Check sheet for the modelled part. Datum: model origin and axes. Units: mm. Give positions to 0.01 mm unless a question says otherwise; leave off trailing zeros. Loops run counter-clockwise (first coordinate to the right, second up) from the corner with the lowest first, then second, coordinate; pieces in that order, holes last. Notation, with made-up numbers: M 45.25,-23.5 L 102.25,-23.5 A29 cw 102.25,2.5 Z; hole C 85.25,37 d7. An arc over 180 degrees is marked long. Write each question's results on one line, items separated by ' | '. Start each with the question number.
1. Sectioned sample at A-A on x = 0. Record the cut outline in (y, z), and give its area (3 significant figures).
2. Draft check along Y on faces 1 (the cylindrical face through (68.86, 21.69, 2.96)), 2 (the flat face through (-1, 1, 0)), 3 (the conical face through (-0.72, 53.74, 3.19)). Enter one of: pulls with the +Y half, pulls with the -Y half, needs draft (parallel to the pull), parting line crosses it, or undercut.
3. Go/stop test with flat-tipped pins: pin 1 (2 mm diameter, centred on x = -32, z = 1.5, fed in from +Y); pin 2 (1.5 mm diameter, centred on y = 54, z = 1, fed in from -X); pin 3 (1.5 mm diameter, centred on x = 16.5, z = 2.5, fed in from -Y); pin 4 (5 mm diameter, centred on x = 0, y = 57, fed in from -Z). Record where each tip stops, or that it passes through.
4. Sectioned sample at C-C on z = 4.8. Record the cut outline in (x, y).
5. Material ranges on line 1 along Y through (x, z) = (0, 2.15); line 2 along Y through (x, z) = (-5, 5.5); line 3 along X through (y, z) = (-35, 5.6), recorded low to high.
6. Sectioned sample at B-B on y = 57. Record the cut outline in (x, z).
7. Sectioned sample at D-D on x = -48. Record the cut outline in (y, z), and give its area (3 significant figures).
```python
from build123d import *

# Parameters (mm, degrees)
F0_R     = 24.06525
F0_R_2   = 1.05
F1_DEPTH = 2
F2_SIZE  = 1
F3_SCALE = 3


with BuildPart() as f1:
    # F0 (on Top) → F1 (new body)
    with BuildSketch(Plane.XY):
        Circle(F0_R)
        with Locations((0, -19)):
            Circle(F0_R_2, mode=Mode.SUBTRACT)
        with Locations((0, 19)):
            Circle(F0_R_2, mode=Mode.SUBTRACT)
    extrude(amount=F1_DEPTH)

    # F2
    f2_edges = [f1.edges().sort_by_distance(p)[0] for p in [
        (-1.05, 19, 2),
        (-1.05, -19, 2),
    ]]
    chamfer(f2_edges, length=F2_SIZE)


with BuildPart() as f1_1:
    # F3: moved
    add(f1.part.scale(F3_SCALE))


solid = f1_1.part
```
Output values:
1) outline: M -72.2,0 L -60.15,0 L -60.15,3 L -63.15,6 L -72.2,6 Z; M -53.85,0 L 53.85,0 L 53.85,3 L 50.85,6 L -50.85,6 L -53.85,3 Z; M 60.15,0 L 72.2,0 L 72.2,6 L 63.15,6 L 60.15,3 Z | area: 773 mm2
2) face 1: parting line crosses it | face 2: needs draft | face 3: undercut
3) pin 1: y = 65.2 | pin 2: x = -48.75 | pin 3: y = -70.46 | pin 4: through
4) outline: C 0,0 d144.39; hole C 0,-57 d9.9; hole C 0,57 d9.9
5) line 1: -72.2 to -60.15, -53.85 to 53.85, 60.15 to 72.2 | line 2: -72.02 to -59.63, -54.37 to 54.37, 59.63 to 72.02 | line 3: -63.14 to 63.14
6) outline: M -44.31,0 L -3.15,0 L -3.15,3 L -6.15,6 L -44.31,6 Z; M 3.15,0 L 44.31,0 L 44.31,6 L 6.15,6 L 3.15,3 Z
7) outline: M -53.93,0 L 53.93,0 L 53.93,6 L -53.93,6 Z | area: 647 mm2
